Read the model definition and answer for the solid it produces. Units are mm, in the model's axes. Face numbers are marked on the shaded views. Give positions to 0.01 mm unless a question says otherwise; leave off trailing zeros. Write each loop counter-clockwise with the first axis right and the second up, starting at its lowest first coordinate (ties: lowest second). Pieces come first, ordered by that corner, then holes. Notation, with made-up numbers: (72, -14) -> (118, -14) arc R7 cw to (118, -4) -> close; hole circle Ø1 at (-30.75, 76.5). An arc over 180 degrees is marked (long way). Use a Markdown table: item, result.
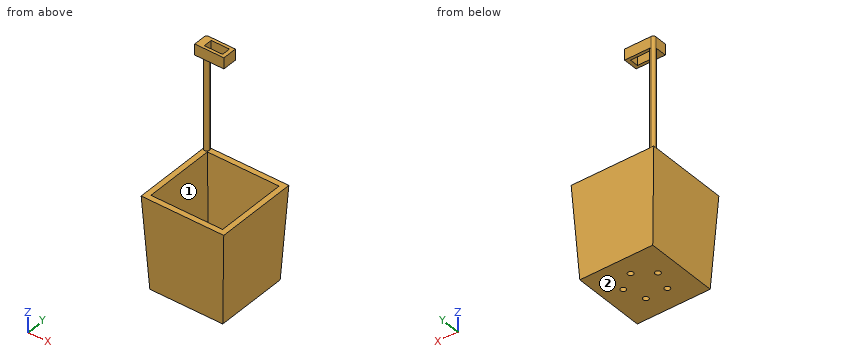
from build123d import *

# Parameters (mm, degrees)
F0_W     = 20
F0_H     = 20
F1_DEPTH = 25.4
F1_TAPER = -3
F2_T     = -1.5
F3_R     = 0.75
F4_DEPTH = 1.5010001
F6_DEPTH = 30
F7_W     = 5
F7_H     = 2.4
F8_DEPTH = 3


with BuildPart() as f1:
    # F0 (on Top) → F1 (new body)
    with BuildSketch(Plane.XY):
        Rectangle(F0_W, F0_H)
    extrude(amount=F1_DEPTH, taper=F1_TAPER)

    # F2
    f2_openings = [f1.faces().sort_by_distance(p)[0] for p in [
        (0, 0, 25.4),
    ]]
    offset(amount=F2_T, openings=f2_openings)

    # F3 (on face) → F4 (cut, through all)
    with BuildSketch(Plane.XY.offset(1.5)):
        with Locations((0, 5)):
            Circle(F3_R)
        with Locations((4.7552825815, 1.5450849719)):
            Circle(F3_R)
        with Locations((2.9389262615, -4.0450849719)):
            Circle(F3_R)
        with Locations((-2.9389262615, -4.0450849719)):
            Circle(F3_R)
        with Locations((-4.7552825815, 1.5450849719)):
            Circle(F3_R)
    extrude(amount=-F4_DEPTH, mode=Mode.SUBTRACT)

    # F5 (on face) → F6 (join)
    with BuildSketch(Plane.XY.offset(25.4)):
        with BuildLine():
            ThreePointArc((-11.3311575938, 10.5801283388), (-10.5801283366, 9.8290990748), (-9.8290990748, 10.5801283343))
            ThreePointArc((-9.8290990748, 10.5801283343), (-10.049070452, 11.1111862166), (-10.5801283343, 11.3311575938))
            ThreePointArc((-10.5801283343, 11.3311575938), (-11.111186215, 11.1111862181), (-11.3311575938, 10.5801283388))
        make_face()
    extrude(amount=F6_DEPTH)

    # F7 (on face) → F8 (join)
    with BuildSketch(Plane.XY.offset(55.4)):
        with BuildLine():
            Line((-3.3311575938, 11.3311575938), (-10.5801283343, 11.3311575938))
            ThreePointArc((-10.5801283343, 11.3311575938), (-10.049070452, 11.1111862166), (-9.8290990748, 10.5801283343))
            ThreePointArc((-9.8290990748, 10.5801283343), (-10.5801283343, 9.8290990748), (-11.3311575938, 10.5801283343))
            Line((-11.3311575938, 10.5801283343), (-11.3311575938, 7.3311575938))
            Line((-11.3311575938, 7.3311575938), (-3.3311575938, 7.3311575938))
            Line((-3.3311575938, 7.3311575938), (-3.3311575938, 11.3311575938))
        make_face()
        with Locations((-6.8311575938, 9.3311575938)):
            Rectangle(F7_W, F7_H, mode=Mode.SUBTRACT)
    extrude(amount=-F8_DEPTH)


solid = f1.part
Item 1: A cutting plane is placed at A-A (z = 41). Give the vertices of the cut face in (x, y), then the cut area to 3 significant figures.
Return value:
| item | result |
|---|---|
| outline | circle Ø1.5 at (-10.58, 10.58) |
| area | 1.77 mm^2 |
Item 2: Straight lines are drawn through the part: line 1 along Z through (x, y) = (2.5, -2.5); line 2 along X through (y, z) = (-8.25, 18.5); line 3 along X through (y, z) = (5.75, 17). For each, find the intervals that lie inside material, in ascending order. Write a range as [from, to].
Return value:
| item | result |
|---|---|
| line 1 | [0, 1.5] |
| line 2 | [-10.97, -9.47], [9.47, 10.97] |
| line 3 | [-10.89, -9.39], [9.39, 10.89] |
Item 3: Each of these flat-tipped pins is pushed along its axis until it touches: P1, Ø8, axis at x = 5, z = 12.5, coming from the +Y side; P2, Ø2.5, axis at x = -6, z = 53.5, coming from the -Y side; P3, Ø5, axis at x = -8.5, y = 1.5, coming from the +Z side. Where does it stop, or does it pass through?
Return value:
| item | result |
|---|---|
| P1 | y = 10.86 |
| P2 | y = 7.33 |
| P3 | z = 25.4 |
Item 4: For a pull along X with two mould halves and no side action, classify the marked faces 1 and 2 as +X half, -X half, draft (parallel to the pull), parting line (faces both ways), or undercut.
Return value:
| item | result |
|---|---|
| face 1 | undercut |
| face 2 | draft |
